```python
from build123d import *

# Parameters (mm, degrees)
SKETCH_W   = 180
SKETCH_H   = 180
SKETCH_W_2 = 150
SKETCH_H_2 = 150
PAD_DEPTH  = 2


with BuildPart() as part:
    # Sketch (on DatumPlane) → Pad (new body)
    with BuildSketch(Plane.XY.offset(-2)):
        Rectangle(SKETCH_W, SKETCH_H)
        Rectangle(SKETCH_W_2, SKETCH_H_2, mode=Mode.SUBTRACT)
    extrude(amount=PAD_DEPTH)


solid = part.part
```
Input: part model. Units: mm. Frame: model coordinates. Coordinates: 2 decimals unless noted, no trailing zeros. Write each loop counter-clockwise with the first axis right and the second up, starting at its lowest first coordinate (ties: lowest second). Pieces come first, ordered by that corner, then holes.
1) Section A-A on x = 5. Output: boundary loops of the cut face in (y, z), and give its area (3 significant figures).
2) Material intervals for line 1 along Y through (x, z) = (12.5, -1.25), sorted ascending.
3) Section B-B on z = -1.35. Output: boundary loops of the cut face in (x, y).
Check result:
1. outline: (-90, -2) - (-75, -2) - (-75, 0) - (-90, 0) - close; (75, -2) - (90, -2) - (90, 0) - (75, 0) - close
1. area: 60.0 mm2
2. line 1: y = -90 to -75, 75 to 90
3. outline: (-90, -90) - (90, -90) - (90, 90) - (-90, 90) - close; hole (-75, -75) - (75, -75) - (75, 75) - (-75, 75) - close
